Read the model definition and answer for the solid it produces. Units are mm, in the model's axes. A direction names the side the tool comes from. Give positions to 0.01 mm unless a question says otherwise; leave off trailing zeros. Write each loop counter-clockwise with the first axis right and the second up, starting at its lowest first coordinate (ties: lowest second). Pieces come first, ordered by that corner, then holes.
```python
from build123d import *

# Parameters (mm, degrees)
F1_DEPTH  = 9
F2_R      = 8
F4_DEPTH  = 25
F5_W      = 120
F5_H      = 9
F6_DEPTH  = 10
F7_W      = 10
F7_H      = 9
F8_DEPTH  = 9
F10_DEPTH = 25


with BuildPart() as f1:
    # F0 (on Top) → F1 (new body)
    with BuildSketch(Plane.XY):
        Polygon((60, 34.6410161514), (-60, 34.6410161514), (0, -69.2820323028), align=None)
    extrude(amount=F1_DEPTH)

    # F2
    f2_edges = [f1.edges().sort_by_distance(p)[0] for p in [
        (0, -69.282032, 4.5),
    ]]
    fillet(f2_edges, radius=F2_R)

    # F3 (on face) → F4 (cut)
    with BuildSketch(Plane.XY.offset(9)):
        with BuildLine():
            Line((11.5, 13.3397459622), (23.5, 13.3397459622))
            ThreePointArc((23.5, 13.3397459622), (17.5, 19.3397459622), (11.5, 13.3397459622))
        make_face()
        with BuildLine():
            ThreePointArc((-23.5, 13.3397459622), (-17.5, 7.3397459622), (-11.5, 13.3397459622))
            Line((-11.5, 13.3397459622), (-23.5, 13.3397459622))
        make_face()
        with BuildLine():
            Line((-23.5, 13.3397459622), (-11.5, 13.3397459622))
            ThreePointArc((-11.5, 13.3397459622), (-17.5, 19.3397459622), (-23.5, 13.3397459622))
        make_face()
        with BuildLine():
            ThreePointArc((11.5, 13.3397459622), (17.5, 7.3397459622), (23.5, 13.3397459622))
            Line((23.5, 13.3397459622), (11.5, 13.3397459622))
        make_face()
    extrude(amount=-F4_DEPTH, mode=Mode.SUBTRACT)

    # F5 (on face) → F6 (cut)
    with BuildSketch(Plane(origin=(0, 34.6410161514, 0), x_dir=(-1, 0, 0), z_dir=(0, 1, 0))):
        with Locations((0, 4.5)):
            Rectangle(F5_W, F5_H)
    extrude(amount=-F6_DEPTH, mode=Mode.SUBTRACT)

    # F7 (on face) → F8 (join)
    with BuildSketch(Plane(origin=(0, 24.6410161514, 0), x_dir=(-1, 0, 0), z_dir=(0, 1, 0))):
        with Locations((-30, 4.5)):
            Rectangle(F7_W, F7_H)
        with Locations((30, 4.5)):
            Rectangle(F7_W, F7_H)
    extrude(amount=F8_DEPTH)

    # F9 (on face) → F10 (cut)
    with BuildSketch(Plane.XY.offset(9)):
        with BuildLine():
            ThreePointArc((2.5, 13.3397459622), (0, 15.8397459622), (-2.5, 13.3397459622))
            Line((-2.5, 13.3397459622), (2.5, 13.3397459622))
        make_face()
        with BuildLine():
            Line((2.5, 13.3397459622), (-2.5, 13.3397459622))
            ThreePointArc((-2.5, 13.3397459622), (0, 10.8397459622), (2.5, 13.3397459622))
        make_face()
    extrude(amount=-F10_DEPTH, mode=Mode.SUBTRACT)


solid = f1.part
```
Item 1: Each of these flat-tipped pins is pushed along its axis until it touches: pin 1 Ø3 at (y, z) = (-11.5, 2) entering from -X; pin 2 Ø7 at (x, y) = (-17.5, 13.34) entering from +Z; pin 3 Ø2.5 at (y, z) = (28.5, 4) entering from -X; pin 4 Ø2.5 at (x, z) = (6.5, 3.5) entering from +Y. Where does it stop, or does it pass through?
Result set:
pin 1: stops at x = -34.23
pin 2: passes through
pin 3: stops at x = -35
pin 4: stops at y = 24.64
Item 2: Section A-A (y = 27) is taken. Write down the section's boundary in (x, z).
Result set:
outline: (-35, 0) - (-25, 0) - (-25, 9) - (-35, 9) - close; (25, 0) - (35, 0) - (35, 9) - (25, 9) - close
Item 3: Which of the six approach directions +Z, -Z, +X, -X, +Y, -Y give full straight-line access (tool end or side, diameter ignored) to faces 5 (the flat face through (0, 24.641, 5)), 6 (the flat face through (-35, 29, 4)), 7 (the flat face through (35, 29, 4))?
Result set:
face 5: +Z, -Z, +Y
face 6: +Z, -Z, -X, +Y
face 7: +Z, -Z, +X, +Y
Item 4: Find the intervals of material crossed by line 1 along X through (y, z) = (27.5, 3); line 2 along X through (y, z) = (14, 3.5); line 3 along Y through (x, z) = (-17.5, 3), in increasing order.
Result set:
line 1: x = -35 to -25, 25 to 35
line 2: x = -48.08 to -23.46, -11.54 to -2.41, 2.41 to 11.54, 23.46 to 48.08
line 3: y = -38.97 to 7.34, 19.34 to 24.64
Item 5: Determine the mould class of faces 1 (the flat face through (25, 29, 4)), 2 (the flat face through (-1, -3, 0)), 3 (the flat face through (30.25, -16.89, 4.44)), 4 (the cylindrical face through (-18.801, 7.482, 4.563)) for opening direction X: pulls with the +X half, pulls with the -X half, needs draft (parallel to the pull), parting line crosses it, or undercut.
Result set:
face 1: undercut
face 2: needs draft
face 3: pulls with the +X half
face 4: undercut
Item 6: Section B-B (x = 0) is taken. Write down the section's boundary in (y, z).
Result set:
outline: (-61.28, 0) - (10.84, 0) - (10.84, 9) - (-61.28, 9) - close; (15.84, 0) - (24.64, 0) - (24.64, 9) - (15.84, 9) - close
Item 7: Section C-C (z = 3) is taken. Write down the section's boundary in (x, y), and give its area (3 significant figures).
Result set:
outline: (-54.23, 24.64) - (-6.93, -57.28) arc R8 ccw to (6.93, -57.28) - (54.23, 24.64) - (35, 24.64) - (35, 33.64) - (25, 33.64) - (25, 24.64) - (-25, 24.64) - (-25, 33.64) - (-35, 33.64) - (-35, 24.64) - close; hole circle Ø12 at (-17.5, 13.34); hole circle Ø5 at (0, 13.34); hole circle Ø12 at (17.5, 13.34)
area: 4,980 mm2
Item 8: Section D-D (y = 17) is taken. Write down the section's boundary in (x, z).
Result set:
outline: (-49.81, 0) - (-22.25, 0) - (-22.25, 9) - (-49.81, 9) - close; (-12.75, 0) - (12.75, 0) - (12.75, 9) - (-12.75, 9) - close; (22.25, 0) - (49.81, 0) - (49.81, 9) - (22.25, 9) - close
